Autodesk Inventor part; units mm, degrees
ref_plane "YZ Plane" through (0, 0, 0) normal (1, 0, 0) x (0, 1, 0)
ref_plane "XZ Plane" through (0, 0, 0) normal (0, 1, 0) x (-1, 0, 0)
ref_plane "XY Plane" through (0, 0, 0) normal (0, 0, 1) x (1, 0, 0)
sketch "Sketch1" plane through (0, 0, 0) normal (0, 1, 0) x (-1, 0, 0)
  line L0 (5.7156, 18.4944) -> (5.7156, 10.6944)
  line L1 (5.7156, 10.6944) -> (-5.2844, 10.6944)
  line L2 (-5.2844, 10.6944) -> (-5.2844, 18.4944)
  line L3 (-5.2844, 18.4944) -> (5.7156, 18.4944)
  point P0 (0, 0)
  dimension "d3" = 7.8
  dimension "d4" = 11
  dimension "d5" = 7.8
  dimension "d6" = 11
extrude "Extrusion1" add sketch "Sketch1" along normal blind 2.8
sketch "Sketch2" plane through (5.2844, 0, 18.4944) normal (1, 0, 0) x (0, 0, -1)
  circle A0 centre (1.263, 1.3452) radius 0.3
  point P0 (18.4944, 0)
  dimension "d10" = 0.6
extrude "Extrusion2" add sketch "Sketch2" along normal blind 16.5
sketch "Sketch3" plane through (5.2844, 0, 18.4944) normal (1, 0, 0) x (0, 0, -1)
  circle A0 centre (1.263, 1.3452) radius 0.3
  line L0 (1.263, 1.3452) -> (3.763, 1.3452)
  circle A1 centre (3.763, 1.3452) radius 0.3
  point P0 (18.4944, 0)
  dimension "d13" = 2.5
  dimension "d14" = 0.6
extrude "Extrusion3" add sketch "Sketch3" along normal blind 16.5 contours A1
sketch "Sketch4" plane through (5.2844, 0, 18.4944) normal (1, 0, 0) x (0, 0, -1)
  circle A0 centre (3.763, 1.3452) radius 0.3
  line L0 (3.763, 1.3452) -> (6.263, 1.3452)
  circle A1 centre (6.263, 1.3452) radius 0.3
  point P0 (18.4944, 0)
  dimension "d17" = 2.5
  dimension "d18" = 0.6
extrude "Extrusion4" add sketch "Sketch4" along normal blind 16.5 contours A1
sketch "Sketch6" plane through (0, 2.8, 0) normal (0, 1, 0) x (1, 0, 0)
  circle A0 centre (0, -14.4314) radius 1.5
  point P0 (0, 0)
hole "Hole1" at (0, 2.8, 14.4314) direction (0, -1, 0) diameter 3 end through all
properties part number "Transistor" material "Copper, Alloy"
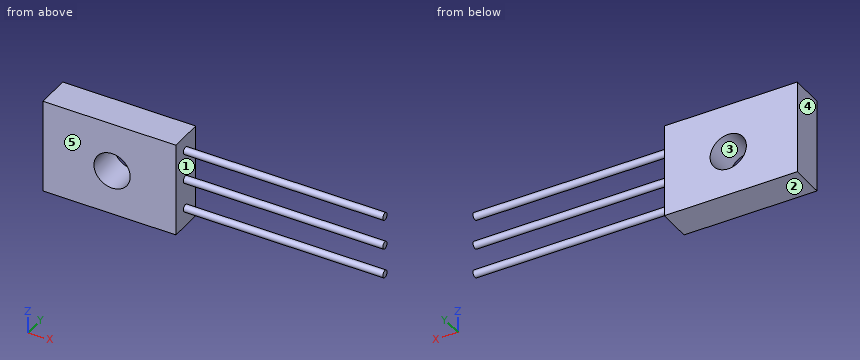
Geometry: final body of the model. Coordinates: model frame, mm. Face numbers are marked on the shaded views. A direction names the side the tool comes from. Coordinates: 2 decimals unless noted, no trailing zeros. Order: outer loops, then holes, each group sorted by start corner. A loop starts at its lowest first (then second) coordinate and runs counter-clockwise, first axis right, second up. Notation, with made-up numbers: M 39.25,14.25 L 96.25,14.25 A16 ccw 96.25,21.25 Z; hole C 62,-31.5 d9. An arc over 180 degrees is marked long. Answer in a Markdown table with one row per item. Add a question column.
Q1. Mould query, pull axis X, two halves, no side actions, for the marked faces 3, 4 and 5. Classes: released by +X, released by -X, zero draft, split by the parting line, or undercut.
Q2. Section query A-A on y = 0.3. Return the cut outline in (x, z), and give its area (3 significant figures).
Q3. Section query C-C on z = 13.25. Return the cut outline in (x, y).
Q4. Section query B-B on x = 0.5. Return the cut outline in (y, z).
Q5. Section query D-D on z = 16.5. Return the cut outline in (x, y).
Q6. Line query: L1, parallel to X at y = 1.4, z = 14.5; L2, parallel to Z at x = 7.5, y = 1.4; L3, parallel to Z at x = 20.25, y = 1.6. Output: solid intervals per line, ascending.
Q7. Reachability of the marked faces 1 and 2 from +Z, -Z, +X, -X, +Y, -Y: full face, straight path, thin tool, end or side. Return the list, or none.
Completed:
| question | item | result |
|---|---|---|
| 1 | face 3 | undercut |
| 1 | face 4 | released by -X |
| 1 | face 5 | zero draft |
| 2 | outline | M -5.72,10.69 L 5.28,10.69 L 5.28,18.49 L -5.72,18.49 Z; hole C 0,14.43 d3 |
| 2 | area | 78.7 mm2 |
| 3 | outline | M -5.72,0 L -0.92,0 L -0.92,2.8 L -5.72,2.8 Z; M 0.92,0 L 5.28,0 L 5.28,2.8 L 0.92,2.8 Z |
| 4 | outline | M 0,10.69 L 2.8,10.69 L 2.8,13.02 L 0,13.02 Z; M 0,15.85 L 2.8,15.85 L 2.8,18.49 L 0,18.49 Z |
| 5 | outline | M -5.72,0 L 5.28,0 L 5.28,2.8 L -5.72,2.8 Z |
| 6 | L1 | x = -5.72 to -1.5, 1.5 to 21.78 |
| 6 | L2 | z = 11.94 to 12.53, 14.44 to 15.03, 16.94 to 17.53 |
| 6 | L3 | z = 12.07 to 12.39, 14.57 to 14.89, 17.07 to 17.39 |
| 7 | face 1 | +X |
| 7 | face 2 | -Z, +X, -X, +Y, -Y |
